The drawing under review shows one solid part. Ordinate dimensions are in mm from its lowest x, y, z. Coordinates: 2 decimals unless noted, no trailing zeros. Loops run counter-clockwise (first coordinate to the right, second up) from the corner with the lowest first, then second, coordinate; pieces in that order, holes last. Notation, with made-up numbers: M 30,70.5 L 44,70.5 A22 ccw 44,93.5 Z; hole C 0.5,-37 d3. An arc over 180 degrees is marked long. Answer as a JSON object with one key per item and string values. Group by question number.
1. Insertion check: pin 1 (1.5 mm diameter, centred on y = 98, z = 1.5, fed in from -X). The pin has a flat end and moves straight along its axis. Give the tip position at first contact, or say it passes through.
2. To check wall thickness, follow probe 1 along X at (y, z) = (47, 0.95). State the ranges of the line that lie inside material, in increasing order.
3. Consider section B-B (y = 117.5). State the section outline as (x, z) points, then the cut area to 3 significant figures.
4. Draft analysis for pull direction Z (two halves, no side actions). For the marked faces 1 and 2, state which applies: +Z half, -Z half, draft (parallel to the pull), parting line (faces both ways), or undercut.
5. Consider section A-A (z = 2.35). State the section outline as (x, y) points, then the cut area to 4 significant figures.
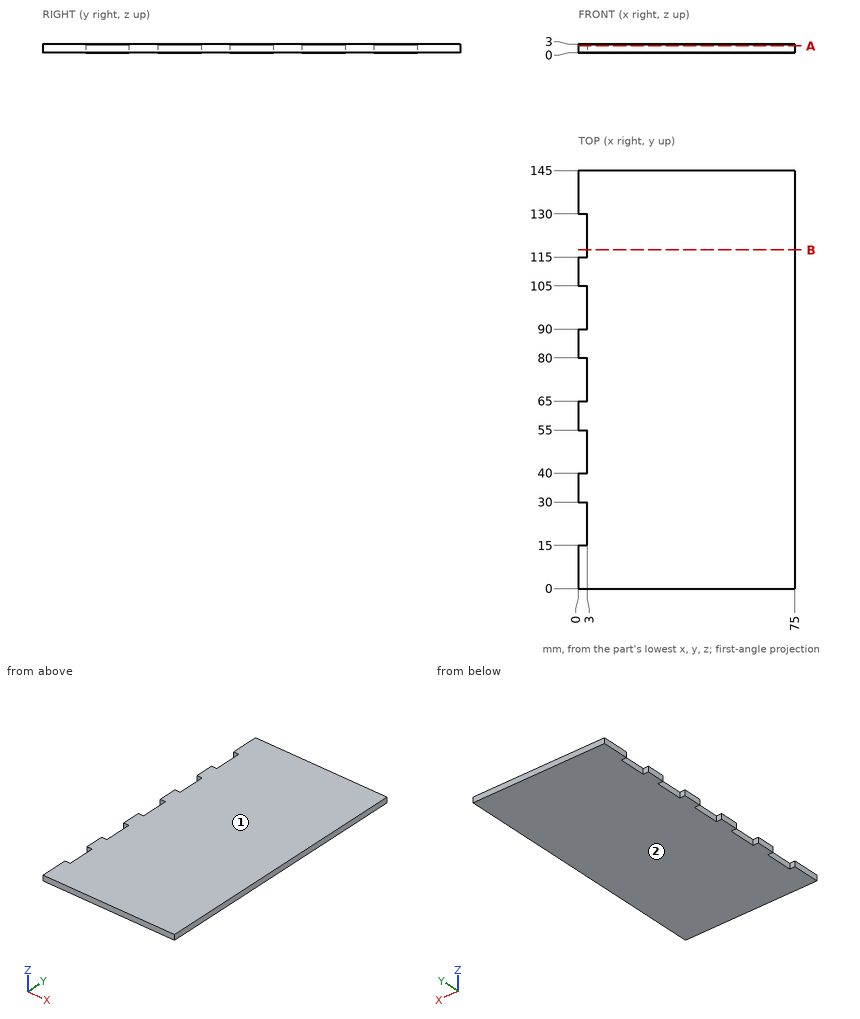
Findings below:
{
 "1": {"pin 1": "stops at x = 3"},
 "2": {"probe 1": "x = 3 to 75"},
 "3": {"outline": "M 3,0 L 75,0 L 75,3 L 3,3 Z", "area": "216 mm^2"},
 "4": {"face 1": "+Z half", "face 2": "-Z half"},
 "5": {"outline": "M 0,0 L 75,0 L 75,145 L 0,145 L 0,130 L 3,130 L 3,115 L 0,115 L 0,105 L 3,105 L 3,90 L 0,90 L 0,80 L 3,80 L 3,65 L 0,65 L 0,55 L 3,55 L 3,40 L 0,40 L 0,30 L 3,30 L 3,15 L 0,15 Z", "area": "10,650 mm^2"}
}
